Can you work these out from the model? Positions are in its coordinate system, mm. A direction names the side the tool comes from. Give positions to 0.01 mm unless a question says otherwise; leave off trailing zeros. Order: outer loops, then holes, each group sorted by start corner. A loop starts at its lowest first (then second) coordinate and runs counter-clockwise, first axis right, second up.
Autodesk Inventor part; units mm, degrees
ref_plane "YZ Plane" through (0, 0, 0) normal (1, 0, 0) x (0, 1, 0)
ref_plane "XZ Plane" through (0, 0, 0) normal (0, 1, 0) x (-1, 0, 0)
ref_plane "XY Plane" through (0, 0, 0) normal (0, 0, 1) x (1, 0, 0)
sketch "Sketch1" plane through (0, 0, 0) normal (0, 1, 0) x (-1, 0, 0)
  line L0 (122.8458, -138.2757) -> (56.882, -138.2757)
  line L1 (56.882, -138.2757) -> (56.882, -265.2757)
  line L2 (56.882, -265.2757) -> (122.8458, -265.2757)
  line L3 (122.8458, -265.2757) -> (122.8458, -138.2757)
  line L4 (110.1458, -173.9373) -> (69.582, -173.9373)
  line L5 (69.582, -173.9373) -> (69.582, -229.6141)
  line L6 (69.582, -229.6141) -> (110.1458, -229.6141)
  line L7 (110.1458, -229.6141) -> (110.1458, -173.9373)
  point P0 (0, 0)
  dimension "d1" = 127
  dimension "d4" = 55.6768
  dimension "d5" = 40.5638
  dimension "d6" = 12.7
  dimension "d7" = 35.6616
  dimension "d8" = 12.7
extrude "Extrusion1" add sketch "Sketch1" along normal blind 63.5 contours L3 L2 L1 L0 | L7 L6 L5 L4
shell "Shell1" thickness 2.54 removed faces 1 at (-56.882, 21.1667, -180.609)
sketch "Sketch3" plane through (0, 63.5, 0) normal (0, 1, 0) x (1, 0, 0)
  line L0 (-110.1458, 174.0389) -> (-69.582, 174.0389)
  line L1 (-69.582, 174.0389) -> (-69.582, 229.7157)
  line L2 (-69.582, 229.7157) -> (-110.1458, 229.7157)
  line L3 (-110.1458, 229.7157) -> (-110.1458, 174.0389)
  line L4 (-122.8458, 265.2757) -> (-122.8458, 138.2757)
  line L5 (-56.882, 265.2757) -> (-122.8458, 265.2757)
  point P0 (0, 0)
  dimension "d14" = 55.6768
  dimension "d15" = 40.5638
  dimension "d16" = 12.7
  dimension "d17" = 35.56
extrude "Extrusion2" cut sketch "Sketch3" against normal blind 12.7
sketch "Sketch4" plane through (0, 63.5, 0) normal (0, 1, 0) x (1, 0, 0)
  circle A0 centre (-91.0958, 156.2589) radius 2.4257
  line L0 (-69.582, 174.0389) -> (-110.1458, 174.0389)
  line L1 (-122.8458, 265.2757) -> (-122.8458, 138.2757)
  line L2 (-122.8458, 138.2757) -> (-56.882, 138.2757)
  line L3 (-69.582, 229.7157) -> (-69.582, 174.0389)
  line L4 (-69.582, 174.0389) -> (-110.1458, 174.0389)
  line L5 (-110.1458, 174.0389) -> (-110.1458, 229.7157)
  line L6 (-110.1458, 229.7157) -> (-69.582, 229.7157)
  line L7 (-122.8458, 138.2757) -> (-56.882, 138.2757)
  line L8 (-56.882, 138.2757) -> (-56.882, 265.2757)
  line L9 (-56.882, 265.2757) -> (-122.8458, 265.2757)
  line L10 (-122.8458, 265.2757) -> (-122.8458, 138.2757)
  circle A1 centre (-91.0958, 247.4957) radius 2.4257
  point P0 (0, 0)
  dimension "d20" = 4.8514
  dimension "d21" = 17.78
  dimension "d22" = 31.75
  dimension "d23" = 4.8514
  dimension "d24" = 17.78
  dimension "d25" = 31.75
hole "Hole1" at (-91.0958, 63.5, -156.2589) at (-91.0958, 63.5, -247.4957) direction (0, -1, 0) diameter 4.8514 depth 12.7 tip angle 118
sketch "Sketch5" plane through (0, 0, 0) normal (0, -1, 0) x (1, 0, 0)
  line L0 (-122.8458, -265.2757) -> (-122.8458, -138.2757)
  line L1 (-122.8458, -138.2757) -> (-56.882, -138.2757)
  line L2 (-122.8458, -265.2757) -> (-122.8458, -138.2757)
  line L3 (-56.882, -265.2757) -> (-122.8458, -265.2757)
  line L4 (-56.882, -138.2757) -> (-56.882, -265.2757)
  line L5 (-96.1758, -206.0937) -> (-87.5398, -206.0937)
  line L6 (-87.5398, -206.0937) -> (-87.5398, -197.4577)
  line L7 (-87.5398, -197.4577) -> (-96.1758, -197.4577)
  line L8 (-96.1758, -197.4577) -> (-96.1758, -206.0937)
  circle A0 centre (-91.8578, -191.8951) radius 1.0414
  circle A1 centre (-91.8578, -212.4032) radius 1.0826
  point P0 (0, 0)
  dimension "d33" = 8.636
  dimension "d34" = 8.636
  dimension "d35" = 26.67
  dimension "d36" = 59.182
  dimension "d64" = 2.0828
  dimension "d65" = 5.5626
  dimension "d83" = 127
  dimension "d84" = 8.636
extrude "Extrusion3" cut sketch "Sketch5" against normal blind 12.7 contours L8 L7 L6 L5
sketch "Sketch6" plane through (-122.8458, 0, -265.2757) normal (-1, 0, 0) x (0, 0, 1)
  circle A0 centre (63.5, 50.8) radius 3.556
  line L0 (127, 0) -> (127, 63.5)
  line L1 (0, 63.5) -> (127, 63.5)
  line L2 (116.7244, 19.05) -> (97.1664, 19.05)
  line L3 (97.1664, 19.05) -> (97.1664, 6.35)
  line L4 (97.1664, 6.35) -> (116.7244, 6.35)
  line L5 (116.7244, 6.35) -> (116.7244, 19.05)
  line L6 (0, 0) -> (127, 0)
  point P0 (265.2757, 0)
  dimension "d39" = 7.112
  dimension "d40" = 63.5
  dimension "d41" = 12.7
  dimension "d49" = 12.7
  dimension "d50" = 19.558
  dimension "d51" = 6.35
hole "Hole2" at (-122.8458, 50.8, -201.7757) direction (1, 0, 0) diameter 7.112 depth 12.7 tip angle 118
extrude "Extrusion4" cut sketch "Sketch6" against normal blind 12.7 contours L5 L4 L3 L2
fillet "Fillet1" radius 6.35 2 edges at (-122.8458, 31.75, -265.2757) (-122.8458, 31.75, -138.2757)
sketch "Sketch8" plane through (0, 63.5, 0) normal (0, 1, 0) x (1, 0, 0)
  point P0 (0, 0)
sketch "Sketch9" plane through (0, 63.5, 0) normal (0, 1, 0) x (1, 0, 0)
  point P0 (0, 0)
sketch "Sketch10" plane through (0, 63.5, 0) normal (0, 1, 0) x (1, 0, 0)
  line L0 (-110.1458, 229.7157) -> (-69.582, 229.7157)
  line L1 (-110.1458, 174.0389) -> (-110.1458, 229.7157)
  line L2 (-69.582, 229.7157) -> (-69.582, 174.0389)
  line L3 (-69.582, 174.0389) -> (-110.1458, 174.0389)
  point P0 (0, 0)
  point P1 (-107.301, 232.5605)
  point P2 (-72.4268, 232.5605)
  point P3 (-107.301, 171.1941)
  point P4 (-72.4268, 171.1941)
  dimension "d66" = 2.8448
  dimension "d67" = 2.8448
  dimension "d68" = 2.8448
  dimension "d69" = 2.8448
  dimension "d70" = 2.8448
  dimension "d71" = 2.8448
  dimension "d72" = 2.8448
  dimension "d73" = 2.8448
hole "Hole4" at (-72.4268, 63.5, -232.5605) at (-107.301, 63.5, -171.1941) at (-72.4268, 63.5, -171.1941) at (-107.301, 63.5, -232.5605) direction (0, -1, 0) diameter 2.6416 depth 12.7 tip angle 118
sketch "Sketch11" plane through (0, 0, 0) normal (0, -1, 0) x (1, 0, 0)
  line L0 (-106.285, -214.7297) -> (-82.155, -214.7297)
  line L1 (-82.155, -214.7297) -> (-82.155, -189.3297)
  line L2 (-82.155, -189.3297) -> (-106.285, -189.3297)
  line L3 (-106.285, -189.3297) -> (-106.285, -214.7297)
  line L4 (-96.1758, -206.0937) -> (-96.1758, -197.4577)
  line L5 (-96.1758, -197.4577) -> (-87.5398, -197.4577)
  line L6 (-87.5398, -206.0937) -> (-96.1758, -206.0937)
  point P0 (0, 0)
  point P1 (-104.2022, -191.4125)
  point P2 (-104.2022, -212.6469)
  point P3 (-91.6292, -212.6469)
  point P4 (-91.6292, -191.4125)
  dimension "d81" = 24.13
  dimension "d82" = 25.4
  dimension "d85" = 14.0208
  dimension "d87" = 16.764
  dimension "d88" = 2.0828
  dimension "d89" = 2.0828
  dimension "d90" = 2.0828
  dimension "d91" = 2.0828
  dimension "d92" = 2.0828
  dimension "d93" = 2.0828
  dimension "d95" = 12.573
  dimension "d96" = 12.573
hole "Hole5" at (-104.2022, 0, -212.6469) at (-104.2022, 0, -191.4125) at (-91.6292, 0, -191.4125) at (-91.6292, 0, -212.6469) direction (0, 1, 0) diameter 2.286 depth 12.7 tip angle 118
sketch "Sketch14" plane through (-56.882, 0, -265.2757) normal (0, 0, -1) x (-1, 0, 0)
  line L0 (17.78, 13.2334) -> (10.16, 13.2334)
  line L1 (10.16, 13.2334) -> (10.16, 10.16)
  line L2 (10.16, 10.16) -> (17.78, 10.16)
  line L3 (17.78, 10.16) -> (17.78, 13.2334)
  line L4 (0, 2.54) -> (63.4238, 2.54)
  line L5 (0, 0) -> (0, 63.5)
  point P0 (-56.882, 0)
  dimension "d114" = 7.62
  dimension "d115" = 3.0734
  dimension "d116" = 7.62
  dimension "d117" = 10.16
extrude "Extrusion6" cut sketch "Sketch14" against normal blind 12.7
equation "\"d7\" = -0.5 * d4 + 0.5 * d1"
equation "\"d8\" = d6"
equation "\"d36\" = 0.5 * d83 - 0.5 * d84"
properties part number "maincontrolpackage_third_eye_not_blind"
1) Suppose I cut it at C-C (y = 50.8). Please give me the cut outline in (x, z), and give its area (3 significant figures).
2) We'd pull the mould along Z, two halves only. Please class faces 5 (the face through (-71, 10.16, -264)), 6 (the face through (-96.176, 1, -202)), 7 (the face through (-71.921, 62.212, -169.974)), 8 (the face through (-86, 31, -265.276)): +Z half, -Z half, draft (parallel to the pull), parting line (faces both ways), or undercut.
3) Suppose I cut it at D-D (z = -257). Please give me the cut outline in (x, y).
4) I'm going to push flat-ended pins straight in: pin 1 Ø3.5 at (x, z) = (-107.3, -232.56) entering from -Y; pin 2 Ø1 at (y, z) = (49.5, -200) entering from -X; pin 3 Ø19 at (x, z) = (-100, -213) entering from +Y; pin 4 Ø6 at (y, z) = (44.5, -167) entering from +X. Where does each tip first touch, or does it pass through?
5) Suppose I cut it at A-A (z = -177). Please give me the cut outline in (x, y).
6) Which directions (+Z, -Z, +X, -X, +Y, -Y) give clear straight access to the entire face, cutting with the end or side of a thin tool? Please do faces 1 (the face through (-122, 19.05, -158)), 2 (the face through (-106.5, 62.21, -233.61)), 3 (the face through (-67.042, 12, -264)), 4 (the face through (-120.306, 31, -203)).
7) If I drill on line 1 (Z direction, x = -97, y = 23); line 2 (Y direction, x = -67, z = -208); line 3 (X direction, y = 60.5, z = -167), over which ranges is the centre line in solid material (lowest first)?
8) Suppose I cut it at B-B (x = -61.5). Please give me the cut outline in (y, z), and give its area (3 significant figures).
Results:
1. outline: (-122.85, -258.93) arc R6.35 ccw to (-116.5, -265.28) - (-56.88, -265.28) - (-56.88, -262.74) - (-120.31, -262.74) - (-120.31, -205.33) - (-122.85, -205.33) - close; (-122.85, -198.22) - (-120.31, -198.22) - (-120.31, -140.82) - (-56.88, -140.82) - (-56.88, -138.28) - (-116.5, -138.28) arc R6.35 ccw to (-122.85, -144.63) - close
1. area: 609 mm2
2. face 5: draft
2. face 6: undercut
2. face 7: undercut
2. face 8: -Z half
3. outline: (-122.85, 0) - (-56.88, 0) - (-56.88, 2.54) - (-120.31, 2.54) - (-120.31, 60.96) - (-56.88, 60.96) - (-56.88, 63.5) - (-122.85, 63.5) - close
4. pin 1: stops at y = 0
4. pin 2: passes through
4. pin 3: stops at y = 2.54
4. pin 4: stops at x = -120.31
5. outline: (-122.85, 0) - (-56.88, 0) - (-56.88, 2.54) - (-120.31, 2.54) - (-120.31, 60.96) - (-110.15, 60.96) - (-110.15, 63.5) - (-122.85, 63.5) - close; (-69.58, 60.96) - (-56.88, 60.96) - (-56.88, 63.5) - (-69.58, 63.5) - close
6. face 1: +X, -X
6. face 2: +Y
6. face 3: -Z
6. face 4: +X
7. line 1: z = -265.28 to -262.74, -140.82 to -138.28
7. line 2: y = 0 to 2.54, 60.96 to 63.5
7. line 3: x = -122.85 to -120.31
8. outline: (0, -265.28) - (63.5, -265.28) - (63.5, -138.28) - (0, -138.28) - close; hole (2.54, -262.74) - (60.96, -262.74) - (60.96, -140.82) - (2.54, -140.82) - close
8. area: 942 mm2
